from build123d import *

# Parameters (mm, degrees)
SKETCH1_R                   = 1.6
BOSS_EXTRUDE1_DEPTH         = 10.5
FILLET1_R                   = 4
SKETCH4_R                   = 2.8
CUT_EXTRUDE1_DEPTH          = 5.5
CHAMFER3_SIZE               = 0.6
REVOLUCI_N1_ANGLE           = 67.5
REVOLUCI_N1_OTHER_WAY_ANGLE = 67.5
CORTAR_EXTRUIR3_DEPTH       = 1
CORTAR_EXTRUIR4_DEPTH       = 54.537370165
CORTAR_EXTRUIR4_DEPTH_BACK  = 54.537370165
CROQUIS6_W                  = 49.797106802
CROQUIS6_H                  = 15.102267028


with BuildPart() as part:
    # Sketch1 → Boss-Extrude1 (new, symmetric)
    with BuildSketch(Plane.XY):
        with BuildLine():
            Line((-32.5, 10.313318502), (-24.898553401, 10.313318502))
            ThreePointArc((-24.898553401, 10.313318502), (0, 26.95), (24.898553401, 10.313318502))
            Line((24.898553401, 10.313318502), (32.5, 10.313318502))
            Line((32.5, 10.313318502), (32.5, 37))
            Line((32.5, 37), (-32.5, 37))
            Line((-32.5, 37), (-32.5, 10.313318502))
        make_face()
        with Locations(Location((-28, 16, 0), (0, 0, 180))):
            Circle(SKETCH1_R, mode=Mode.SUBTRACT)
        with Locations(Location((-28, 32, 0), (0, 0, 180))):
            Circle(SKETCH1_R, mode=Mode.SUBTRACT)
        with Locations(Location((28, 16, 0), (0, 0, 180))):
            Circle(SKETCH1_R, mode=Mode.SUBTRACT)
        with Locations(Location((0, 32, 0), (0, 0, 180))):
            Circle(SKETCH1_R, mode=Mode.SUBTRACT)
        with Locations(Location((28, 32, 0), (0, 0, 180))):
            Circle(SKETCH1_R, mode=Mode.SUBTRACT)
    extrude(amount=BOSS_EXTRUDE1_DEPTH, both=True)

    # Fillet1
    fillet1_edges = [part.edges().sort_by_distance(p)[0] for p in [
        (-32.5, 10.313318502, 0),
        (-32.5, 37, 0),
        (32.5, 37, 0),
        (32.5, 10.313318502, 0),
    ]]
    fillet(fillet1_edges, radius=FILLET1_R)

    # Sketch4 → Cut-Extrude1 (cut)
    with BuildSketch(Plane(origin=(0, 0, -10.5), x_dir=(-1, 0, 0), z_dir=(0, 0, -1))):
        with Locations((-28, 32)):
            Circle(SKETCH4_R)
        with Locations((0, 32)):
            Circle(SKETCH4_R)
        with Locations((28, 32)):
            Circle(SKETCH4_R)
        with Locations((-28, 16)):
            Circle(SKETCH4_R)
        with Locations((28, 16)):
            Circle(SKETCH4_R)
    extrude(amount=-CUT_EXTRUDE1_DEPTH, mode=Mode.SUBTRACT)

    # Chamfer3
    chamfer3_edges = [part.edges().sort_by_distance(p)[0] for p in [
        (30.8, 16, -10.5),
        (-25.2, 32, -10.5),
        (2.8, 32, -10.5),
        (30.8, 32, -10.5),
    ]]
    chamfer(chamfer3_edges, length=CHAMFER3_SIZE)

    # Croquis1 → Revolución1 (revolve)
    with BuildSketch(Plane(origin=(0, 0, 0), x_dir=(0, 0, -1), z_dir=(1, 0, 0))):
        with BuildLine():
            Line((10.5, 26.95), (-10.5, 26.95))
            Line((-10.5, 26.95), (-10.5, 23.95))
            add(Edge.make_bspline(
                [(10.5, 23.95), (7.13922955, 23.695558229), (0, 30.004441771), (-7.13922955, 23.695558229), (-10.5, 23.95)],
                knots=[0, 0, 0, 0, 0.5, 1, 1, 1, 1], degree=3))
            Line((10.5, 23.95), (10.5, 26.95))
        make_face()
    revolve(axis=Axis((0, 0, 10.5), (0, 0, -1)), revolution_arc=REVOLUCI_N1_ANGLE)

    # Croquis1 → Revolución1 other way (revolve)
    with BuildSketch(Plane(origin=(0, 0, 0), x_dir=(0, 0, -1), z_dir=(1, 0, 0))):
        with BuildLine():
            Line((10.5, 26.95), (-10.5, 26.95))
            Line((-10.5, 26.95), (-10.5, 23.95))
            add(Edge.make_bspline(
                [(10.5, 23.95), (7.13922955, 23.695558229), (0, 30.004441771), (-7.13922955, 23.695558229), (-10.5, 23.95)],
                knots=[0, 0, 0, 0, 0.5, 1, 1, 1, 1], degree=3))
            Line((10.5, 23.95), (10.5, 26.95))
        make_face()
    revolve(axis=Axis((0, 0, 10.5), (0, 0, 1)), revolution_arc=REVOLUCI_N1_OTHER_WAY_ANGLE)

    # Croquis5 → Cortar-Extruir3 (cut)
    with BuildSketch(Plane(origin=(0, 0, -10.5), x_dir=(-1, 0, 0), z_dir=(0, 0, -1))):
        Polygon((-17.822469022, 29.950787399), (-17.11776149, 29.950787399), (-15.408146105, 25.717454066), (-16.219704599, 25.717454066), (-16.548737719, 26.585830134), (-18.393188841, 26.585830134), (-18.72222196, 25.717454066), (-19.53293243, 25.717454066), align=None)
        Polygon((-17.470539268, 28.815283927), (-18.104860849, 27.345659194), (-16.836217687, 27.345659194), align=None, mode=Mode.SUBTRACT)
    extrude(amount=-CORTAR_EXTRUIR3_DEPTH, mode=Mode.SUBTRACT)

    # Croquis6 → Cortar-Extruir4 (cut, two sides: drawn at the far end of the back side and taken through both)
    with BuildSketch(Plane(origin=(0, 0, -10.5), x_dir=(-1, 0, 0), z_dir=(0, 0, -1)).offset(-CORTAR_EXTRUIR4_DEPTH_BACK)):
        with Locations((0, 2.762184988)):
            Rectangle(CROQUIS6_W, CROQUIS6_H)
    extrude(amount=CORTAR_EXTRUIR4_DEPTH + CORTAR_EXTRUIR4_DEPTH_BACK, mode=Mode.SUBTRACT)


solid = part.part
Verification items for the finished model (mm, model axes). A direction names the side the tool comes from. Coordinates: 2 decimals unless noted, no trailing zeros. One line per item, written item: value. Start each with the question number.
Item 1: Mould release check, pull along X, two halves, no side actions. Record for faces 3 (the flat face through (26, 10.313, 0)), 4 (the cylindrical face through (-31.297, 11.454, -0.147)), 5 (the cylindrical face through (29.27, 32.97, 2.64)), 6 (the flat face through (16.275, 27.864, -10.007)): pulls with the +X half, pulls with the -X half, needs draft (parallel to the pull), parting line crosses it, or undercut.
Item 2: Depth check by flat-ended pin: P1, Ø1.7, axis at x = 27.5, y = 31, coming from the -Z side; P2, Ø6.5, axis at x = 28, y = 32, coming from the -Z side. Enter the tip coordinate at first touch or a pass-through.
Item 3: Access from +Z, -Z, +X, -X, +Y, -Y to the whole of each face (thin tool, end or side, straight path). Record for faces 1 (the cylindrical face through (29.18, 14.92, 2.64)), 2 (the cylindrical face through (-25.778, 14.296, -7.788)).
Item 4: Thickness scan on probe 1 along Y at (x, z) = (28, 4.5); probe 2 along Y at (x, z) = (28, -6.75); probe 3 along X at (y, z) = (29.5, -6.25). Record the ranges inside material, lowest first.
Item 5: Sectioned sample at A-A on y = 32. Give the number of separate pieces and of enclosed holes in the cut face, then the cut area to 3 significant figures.
Calculated:
1. face 3: needs draft
1. face 4: pulls with the -X half
1. face 5: undercut
1. face 6: undercut
2. P1: z = -5
2. P2: z = -10.35
3. face 1: +Z, -Z
3. face 2: -Z
4. probe 1: 10.31 to 14.4, 17.6 to 30.4, 33.6 to 37
4. probe 2: 10.31 to 13.2, 18.8 to 29.2, 34.8 to 37
4. probe 3: -32.5 to -29.26, -26.74 to -1.26, 1.26 to 26.74, 29.26 to 32.5
5. separate pieces: 4
5. enclosed holes: 0
5. area: 1,120 mm^2
